Could you check a few things on this model? Use its own coordinates, in mm. A direction names the side the tool comes from. Round coordinates to 2 decimals unless told otherwise and drop trailing zeros. Loops run counter-clockwise (first coordinate to the right, second up) from the corner with the lowest first, then second, coordinate; pieces in that order, holes last.
from build123d import *

# Parameters (mm, degrees)
BOSS_EXTRUDE1_DEPTH = 61
SKETCH2_R           = 3
CUT_EXTRUDE1_DEPTH  = 90.16066958
FILLET1_R           = 5


with BuildPart() as part:
    # Sketch1 → Boss-Extrude1 (new body)
    with BuildSketch(Plane(origin=(0, 0, 0), x_dir=(1, 0, 0), z_dir=(0, 1, 0))):
        with BuildLine():
            Line((-31.75, 0), (-41.75, 0))
            Line((-41.75, 0), (-56.75, 0))
            Line((-56.75, 0), (-56.75, -10))
            Line((-56.75, -10), (-40.534707351, -10))
            ThreePointArc((-40.534707351, -10), (0, -41.75), (40.534707351, -10))
            Line((40.534707351, -10), (56.75, -10))
            Line((56.75, -10), (56.75, 0))
            Line((56.75, 0), (41.75, 0))
            Line((41.75, 0), (31.75, 0))
            ThreePointArc((31.75, 0), (0, -31.75), (-31.75, 0))
        make_face()
    extrude(amount=BOSS_EXTRUDE1_DEPTH)

    # Sketch2 → Cut-Extrude1 (cut, through all)
    with BuildSketch(Plane.XY.offset(10)):
        with Locations((-49.25, 51)):
            Circle(SKETCH2_R)
        with Locations((-49.25, 10)):
            Circle(SKETCH2_R)
        with Locations(Location((49.25, 10, 0), (0, 0, 180))):
            Circle(SKETCH2_R)
        with Locations(Location((49.25, 51, 0), (0, 0, 180))):
            Circle(SKETCH2_R)
    extrude(amount=-CUT_EXTRUDE1_DEPTH, mode=Mode.SUBTRACT)

    # Fillet1
    fillet1_edges = [part.edges().sort_by_distance(p)[0] for p in [
        (40.534707351, 30.5, 10),
        (-40.534707351, 30.5, 10),
    ]]
    fillet(fillet1_edges, radius=FILLET1_R)


solid = part.part
Item 1: If we section it at D-D, the plane y = 39: Please give me the cut outline in (x, z).
Results list:
outline: (-56.75, 0) - (-31.75, 0) arc R31.75 cw to (31.75, 0) - (56.75, 0) - (56.75, 10) - (44.28, 10) arc R5 cw to (39.54, 13.4) arc R41.75 ccw to (-39.54, 13.4) arc R5 cw to (-44.28, 10) - (-56.75, 10) - close
Item 2: For faces 4 (the flat face through (50, 30, 10)), 5 (the cylindrical face through (-52.247, 10.132, 5.07)), 6 (the flat face through (-51, 30, 10)), which set-ups out of +Z, -Z, +X, -X, +Y, -Y let a thin tool reach every point of the face, with its end or its side?
Results list:
face 4: +Z, +X, +Y, -Y
face 5: +Z, -Z
face 6: +Z, -X, +Y, -Y
Item 3: We'd pull the mould along X, two halves only. Please class faces 1 (the cylindrical face through (51.46, 48.97, 5.07)), 2 (the flat face through (-56.75, 30, 5)), 3 (the flat face through (-44, 30, 0)): released by +X, released by -X, zero draft, split by the parting line, or undercut.
Results list:
face 1: undercut
face 2: released by -X
face 3: zero draft
Item 4: If we section it at B-B, the plane x = 49.25: Please give me the cut outline in (y, z), then the cut area to 3 significant figures.
Results list:
outline: (0, 0) - (7, 0) - (7, 10) - (0, 10) - close; (13, 0) - (48, 0) - (48, 10) - (13, 10) - close; (54, 0) - (61, 0) - (61, 10) - (54, 10) - close
area: 490 mm2
Item 5: If we section it at C-C, the plane z = 28: Please give me the cut outline in (x, y), then the cut area to 3 significant figures.
Results list:
outline: (-30.97, 0) - (-14.97, 0) - (-14.97, 61) - (-30.97, 61) - close; (14.97, 0) - (30.97, 0) - (30.97, 61) - (14.97, 61) - close
area: 1,950 mm2
Item 6: If I drill on line 1 along Y through (x, z) = (49.25, 7.25); line 2 along Y through (x, z) = (48, 3.5); line 3 along Z through (x, y) = (48, 23.5), over which ranges is the centre line in solid material (lowest first)?
Results list:
line 1: y = 0 to 7, 13 to 48, 54 to 61
line 2: y = 0 to 7.27, 12.73 to 48.27, 53.73 to 61
line 3: z = 0 to 10
Item 7: Will these pins go through, and if not, where does the flat tip stop? pin 1 (6 mm diameter, centred on x = -49.5, y = 44, fed in from +Z); pin 2 (1.5 mm diameter, centred on x = 11, y = 31, fed in from -Z); pin 3 (12 mm diameter, centred on x = 40, y = 50.5, fed in from +Z).
Results list:
pin 1: stops at z = 10
pin 2: stops at z = 29.5
pin 3: stops at z = 24.23
Item 8: If we section it at A-A, the plane y = 51: Please give me the cut outline in (x, z).
Results list:
outline: (-56.75, 0) - (-52.25, 0) - (-52.25, 10) - (-56.75, 10) - close; (-46.25, 0) - (-31.75, 0) arc R31.75 cw to (31.75, 0) - (46.25, 0) - (46.25, 10) - (44.28, 10) arc R5 cw to (39.54, 13.4) arc R41.75 ccw to (-39.54, 13.4) arc R5 cw to (-44.28, 10) - (-46.25, 10) - close; (52.25, 0) - (56.75, 0) - (56.75, 10) - (52.25, 10) - close
